Work out the finished part from the listing and answer in its coordinate system (mm). A direction names the side the tool comes from. Coordinates: 2 decimals unless noted, no trailing zeros. Order: outer loops, then holes, each group sorted by start corner. A loop starts at its lowest first (then second) coordinate and runs counter-clockwise, first axis right, second up. Notation, with made-up numbers: M 51,58 L 84,58 A9 ccw 84,65 Z; hole C 67.5,-30.75 d9. An arc over 180 degrees is marked long. Answer in a Markdown table with one row per item. Add a question column.
Item 1: A flat-ended cylindrical pin translates along its axis: pin 1 Ø1.7 at (x, y) = (10, 21) entering from +Z. Find the tip coordinate at first contact, or state that the pin passes through.
Item 2: The part is cut by section D-D (z = -0.5). State how many separate pieces and enclosed holes the cut face has, then the cut area to 3 significant figures.
Item 3: The part is cut by section B-B (x = 0). Write down the section's boundary in (y, z), then the cut area to 3 significant figures.
Item 4: The mould has two halves that part along Z. Classify faces 1 (the face through (11.93, 57.4, -0.79)), 2 (the face through (0, 29, 0)): released by +Z, released by -Z, zero draft, split by the parting line, or undercut.
Item 5: Which of the six approach directions +Z, -Z, +X, -X, +Y, -Y give full straight-line access (tool end or side, diameter ignored) to faces 3 (the face through (11.9, 41.07, -0.79)), 4 (the face through (11.9, 0.57, -0.79)), 5 (the face through (0, 39.5, -1))?
Item 6: The part is cut by section C-C (x = 9.5). Write down the section's boundary in (y, z), then the cut area to 3 significant figures.
Item 7: Consider line 1 (Y direction, x = -10, z = -0.6); line 2 (Y direction, x = -9.5, z = -0.7); line 3 (Y direction, x = 0, z = -0.15). Determine where each line is inside the solid, lowest interval first. Write a range as from..to.
Item 8: The part is cut by section A-A (y = 21). Write down the section's boundary in (x, z).
from build123d import *

# Parameters (mm, degrees)
PAD_DEPTH       = 1.6
SKETCH001_R     = 0.5
POCKET_DEPTH    = 1.601
SKETCH002_R     = 1.05
POCKET001_DEPTH = 1.601
POCKET002_DEPTH = 1.601


with BuildPart() as part:
    # Sketch → Pad (new body)
    with BuildSketch(Plane.XY):
        with BuildLine():
            Line((-10.5, 0), (10.5, 0))
            ThreePointArc((10.5, 0), (11.914214, 0.585786), (12.5, 2))
            Line((12.5, 2), (12.5, 56))
            ThreePointArc((12.5, 56), (11.914214, 57.414214), (10.5, 58))
            Line((10.5, 58), (-10.5, 58))
            ThreePointArc((-10.5, 58), (-11.914214, 57.414214), (-12.5, 56))
            Line((-12.5, 56), (-12.5, 2))
            ThreePointArc((-12.5, 2), (-11.914214, 0.585786), (-10.5, 0))
        make_face()
    extrude(amount=-PAD_DEPTH)

    # Sketch001 → Pocket (cut, through all)
    with BuildSketch(Plane.XY):
        with Locations((-11.125, 3)):
            Circle(SKETCH001_R)
        with Locations((11.125, 3)):
            Circle(SKETCH001_R)
        with Locations((-11.125, 5.5)):
            Circle(SKETCH001_R)
        with Locations((-11.125, 8)):
            Circle(SKETCH001_R)
        with Locations((-11.125, 10.5)):
            Circle(SKETCH001_R)
        with Locations((-11.125, 13)):
            Circle(SKETCH001_R)
        with Locations((-11.125, 15.5)):
            Circle(SKETCH001_R)
        with Locations((-11.125, 18)):
            Circle(SKETCH001_R)
        with Locations((11.125, 18)):
            Circle(SKETCH001_R)
        with Locations((11.125, 15.5)):
            Circle(SKETCH001_R)
        with Locations((11.125, 13)):
            Circle(SKETCH001_R)
        with Locations((11.125, 10.5)):
            Circle(SKETCH001_R)
        with Locations((11.125, 8)):
            Circle(SKETCH001_R)
        with Locations((11.125, 5.5)):
            Circle(SKETCH001_R)
    extrude(amount=-POCKET_DEPTH, mode=Mode.SUBTRACT)

    # Sketch002 → Pocket001 (cut, through all)
    with BuildSketch(Plane.XY):
        with Locations((-10, 21)):
            Circle(SKETCH002_R)
        with Locations((10, 21)):
            Circle(SKETCH002_R)
        with Locations((10, 56.5)):
            Circle(SKETCH002_R)
        with Locations((-10, 56.5)):
            Circle(SKETCH002_R)
    extrude(amount=-POCKET001_DEPTH, mode=Mode.SUBTRACT)

    # Sketch003 → Pocket002 (cut, through all)
    with BuildSketch(Plane.XY):
        with BuildLine():
            ThreePointArc((-1.75, 40.500236), (-2.250118, 40.000118), (-1.75, 39.5))
            Line((-1.75, 39.5), (1.75, 39.5))
            ThreePointArc((1.75, 39.5), (2.250118, 40.000118), (1.75, 40.500236))
            Line((-1.75, 40.500236), (1.75, 40.500236))
        make_face()
        with BuildLine():
            ThreePointArc((8.75, 40.500236), (8.249882, 40.000118), (8.75, 39.5))
            Line((8.75, 39.5), (10.5, 39.5))
            ThreePointArc((12.5, 37.500001), (11.914213, 38.914214), (10.5, 39.5))
            Line((12.5, 35.000118), (12.5, 37.500001))
            Line((22.5, 35.000118), (12.5, 35.000118))
            Line((22.5, 45.000118), (22.5, 35.000118))
            Line((12.5, 45.000118), (22.5, 45.000118))
            Line((12.5, 42.500236), (12.5, 45.000118))
            ThreePointArc((10.5, 40.500236), (11.914214, 41.086022), (12.5, 42.500236))
            Line((8.75, 40.500236), (10.5, 40.500236))
        make_face()
        with BuildLine():
            ThreePointArc((-8.75, 39.500118), (-8.25, 40.000118), (-8.75, 40.500118))
            Line((-10.5, 40.500118), (-8.75, 40.500118))
            ThreePointArc((-12.5, 42.500118), (-11.914214, 41.085904), (-10.5, 40.500118))
            Line((-12.5, 42.500118), (-12.5, 45.000118))
            Line((-12.5, 45.000118), (-22.5, 45.000118))
            Line((-22.5, 45.000118), (-22.5, 35.000118))
            Line((-22.5, 35.000118), (-12.5, 35.000118))
            Line((-12.5, 35.000118), (-12.5, 37.500118))
            ThreePointArc((-10.5, 39.500118), (-11.914214, 38.914331), (-12.5, 37.500118))
            Line((-10.5, 39.500118), (-8.75, 39.500118))
        make_face()
    extrude(amount=-POCKET002_DEPTH, mode=Mode.SUBTRACT)


solid = part.part
Reply:
| question | item | result |
|---|---|---|
| 1 | pin 1 | passes through |
| 2 | separate pieces | 1 |
| 2 | enclosed holes | 19 |
| 2 | area | 1,410 mm2 |
| 3 | outline | M 0,-1.6 L 39.5,-1.6 L 39.5,0 L 0,0 Z; M 40.5,-1.6 L 58,-1.6 L 58,0 L 40.5,0 Z |
| 3 | area | 91.2 mm2 |
| 4 | face 1 | zero draft |
| 4 | face 2 | released by +Z |
| 5 | face 3 | +Z, -Z, +X |
| 5 | face 4 | +Z, -Z, +X, -Y |
| 5 | face 5 | +Z, -Z |
| 6 | outline | M 0,-1.6 L 20.08,-1.6 L 20.08,0 L 0,0 Z; M 21.92,-1.6 L 39.5,-1.6 L 39.5,0 L 21.92,0 Z; M 40.5,-1.6 L 55.58,-1.6 L 55.58,0 L 40.5,0 Z; M 57.42,-1.6 L 58,-1.6 L 58,0 L 57.42,0 Z |
| 6 | area | 85.3 mm2 |
| 7 | line 1 | y = 0..19.95, 22.05..39.5, 40.5..55.45, 57.55..58 |
| 7 | line 2 | y = 0..20.08, 21.92..39.5, 40.5..55.58, 57.42..58 |
| 7 | line 3 | y = 0..39.5, 40.5..58 |
| 8 | outline | M -12.5,-1.6 L -11.05,-1.6 L -11.05,0 L -12.5,0 Z; M -8.95,-1.6 L 8.95,-1.6 L 8.95,0 L -8.95,0 Z; M 11.05,-1.6 L 12.5,-1.6 L 12.5,0 L 11.05,0 Z |
